```python
from build123d import *

# Parameters (mm, degrees)
SKETCH1_R           = 5
BOSS_EXTRUDE1_DEPTH = 15
CUT_EXTRUDE1_DEPTH  = 17.583123952
SKETCH3_R           = 3.558152216
BOSS_EXTRUDE2_DEPTH = 15
CUT_EXTRUDE3_DEPTH  = 8


with BuildPart() as part:
    # Sketch1 → Boss-Extrude1 (new body)
    with BuildSketch(Plane(origin=(0, 0, 0), x_dir=(1, 0, 0), z_dir=(0, 1, 0))):
        with Locations(Location((0, 0, 0), (0, 0, 270))):
            Circle(SKETCH1_R)
    extrude(amount=BOSS_EXTRUDE1_DEPTH)

    # Sketch2 → Cut-Extrude1 (cut, through all)
    with BuildSketch(Plane(origin=(0, 15, 0), x_dir=(1, 0, 0), z_dir=(0, 1, 0))):
        with BuildLine():
            Line((-2.096780408, 1.361437447), (-2.096780408, -1.361437447))
            ThreePointArc((-2.096780408, -1.361437447), (2.5, 0), (-2.096780408, 1.361437447))
        make_face()
    extrude(amount=-CUT_EXTRUDE1_DEPTH, mode=Mode.SUBTRACT)

    # Sketch3 → Boss-Extrude2 (add)
    with BuildSketch(Plane(origin=(0, 15, 0), x_dir=(1, 0, 0), z_dir=(0, 1, 0))):
        with BuildLine():
            Line((0, 8), (60, 6))
            ThreePointArc((60, 6), (66, 0), (60, -6))
            Line((60, -6), (0, -8))
            ThreePointArc((0, -8), (-8, 0), (0, 8))
        make_face()
        Circle(SKETCH3_R, mode=Mode.SUBTRACT)
    extrude(amount=-BOSS_EXTRUDE2_DEPTH)

    # Sketch5 → Cut-Extrude3 (cut)
    with BuildSketch(Plane(origin=(0, 15, 0), x_dir=(1, 0, 0), z_dir=(0, 1, 0))):
        with BuildLine():
            Line((60, 6), (0.532741398, 7.982241953))
            ThreePointArc((0.532741398, 7.982241953), (8, 0), (0.532741398, -7.982241953))
            Line((0.532741398, -7.982241953), (60, -6))
            ThreePointArc((60, -6), (54, 0), (60, 6))
        make_face()
    extrude(amount=-CUT_EXTRUDE3_DEPTH, mode=Mode.SUBTRACT)


solid = part.part
```
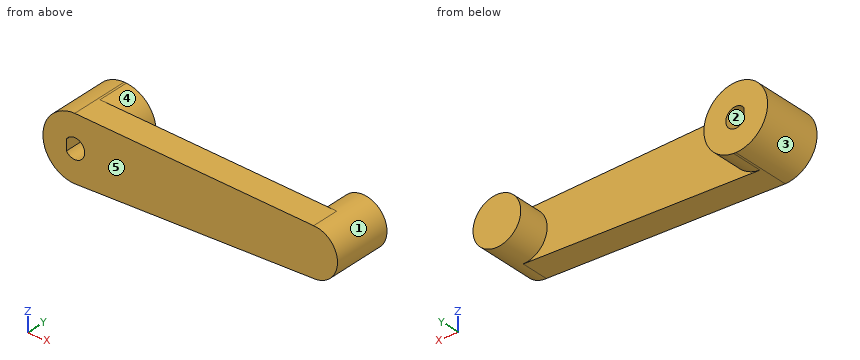
For this review, take the finished solid that the model builds, in its own axes (mm). Face numbers are marked on the shaded views. A direction names the side the tool comes from. Coordinates: 2 decimals unless noted, no trailing zeros. Order: outer loops, then holes, each group sorted by start corner. A loop starts at its lowest first (then second) coordinate and runs counter-clockwise, first axis right, second up. Notation, with made-up numbers: (-29.5, -9) - (-1.5, -9) arc R23 ccw to (-1.5, 13) - close; hole circle Ø2 at (47.5, 34). An arc over 180 degrees is marked (long way). Answer as a JSON object with one key per item and string values. Group by question number.
1. We need section A-A on y = 10.5. State the section outline as (x, z) points, then the cut area to 3 significant figures.
2. For probe 1 along X at (y, z) = (9.5, 0); probe 2 along Z at (x, y) = (0, 11.75); probe 3 along X at (y, z) = (4, 0), list the stretches that pass through material, from the lowest coordinate up.
3. We need section C-C on y = 3. State the section outline as (x, z) points.
4. We need section B-B on z = 0. State the section outline as (x, y) points.
5. We need section D-D on z = -4.25. State the section outline as (x, y) points, then the cut area to 3 significant figures.
6. Clearance check with flat-ended pins moving along their axes: P1, Ø1.5, axis at y = 6, z = 2, coming from the +X side; P2, Ø4, axis at x = 44.5, z = -3, coming from the -Y side; P3, Ø2, axis at x = 42, y = 3.5, coming from the +Z side; P4, Ø8, axis at x = 26, y = 4, coming from the +Z side. State where each tip first meets the part, or that it passes through.
7. The part is to be moulded in two halves that separate along X. For the marked faces 3, 4 and 5, say which applies: pulls with the +X half, pulls with the -X half, needs draft (parallel to the pull), parting line crosses it, or undercut.
8. For the marked faces 1 and 2, list the 3-axis set-ups (+Z, -Z, +X, -X, +Y, -Y) from which the entire face can be reached by the end or side of a thin tool; tool diameter is ignored.
Final values:
{
 "1": {"outline": "(0, -8) - (0.53, -7.98) arc R8 ccw to (0.53, 7.98) - (0, 8) arc R8 ccw to start; circle Ø12 at (60, 0); hole (-2.1, -1.36) arc R2.5 ccw (long way) to (-2.1, 1.36) - close", "area": "295 mm²"},
 "2": {"probe 1": "-8 to -2.1, 2.5 to 8, 54 to 66", "probe 2": "-8 to -2.5, 2.5 to 8", "probe 3": "-8 to -2.1, 2.5 to 66"},
 "3": {"outline": "(0, -8) - (60, -6) arc R6 ccw to (60, 6) - (0, 8) arc R8 ccw to start; hole (-2.1, -1.36) arc R2.5 ccw (long way) to (-2.1, 1.36) - close"},
 "4": {"outline": "(-8, 0) - (-2.1, 0) - (-2.1, 15) - (-8, 15) - close; (2.5, 0) - (66, 0) - (66, 15) - (54, 15) - (54, 7) - (8, 7) - (8, 15) - (2.5, 15) - close"},
 "5": {"outline": "(-6.78, 0) - (64.24, 0) - (64.24, 15) - (55.76, 15) - (55.76, 7) - (6.78, 7) - (6.78, 15) - (-6.78, 15) - close", "area": "673 mm²"},
 "6": {"P1": "x = 65.87", "P2": "y = 0", "P3": "z = 6.63", "P4": "z = 7.27"},
 "7": {"face 3": "pulls with the -X half", "face 4": "undercut", "face 5": "needs draft"},
 "8": {"face 1": "+Y", "face 2": "+Y, -Y"}
}
